Verification items for the finished model (mm, model axes). A direction names the side the tool comes from. Coordinates: 2 decimals unless noted, no trailing zeros. Order: outer loops, then holes, each group sorted by start corner. A loop starts at its lowest first (then second) coordinate and runs counter-clockwise, first axis right, second up. Notation, with made-up numbers: (47, -22.5) -> (105, -22.5) arc R34 ccw to (105, 11.5) -> close; hole circle Ø9 at (-25.5, 41). An arc over 180 degrees is marked (long way). Write each question's results on one line, items separated by ' | '. Start each with the question number.
(1) Go/stop test with flat-tipped pins: pin 1 (1 mm diameter, centred on x = -0.5, z = -1.5, fed in from +Y); pin 2 (11.5 mm diameter, centred on x = 0, z = 0, fed in from -Y); pin 3 (5 mm diameter, centred on x = 6, y = -2, fed in from +Z); pin 4 (5 mm diameter, centred on y = -3.5, z = 2.5, fed in from +X). Record where each tip stops, or that it passes through.
(2) Cross-section at A-A on y = -7.25. Enter the section's corners in (x, z).
(3) Cross-section at C-C on x = 1. Enter the section's corners in (y, z), and give its area (3 significant figures).
(4) Cross-section at B-B on z = 0. Enter the section's corners in (x, y).
(5) Cross-section at D-D on y = -0.25. Enter the section's corners in (x, z), and give its area (3 significant figures).
(6) Thickness scan on probe 1 along Z at (x, y) = (0, 0.1); probe 2 along X at (y, z) = (-7.5, -1.5); probe 3 along Z at (x, y) = (3.5, -5). Record the ranges inside material, lowest first. Write a range as [from, to].
(7) Draft check along X on faces 1 (the flat face through (-14.5, -10.3, 10.4)), 2 (the flat face through (-17.27, -5.48, 5.78)), 3 (the flat face through (8, -0.8, -4)). Enter one of: +X half, -X half, draft (parallel to the pull), parting line (faces both ways), or undercut.
(8) Set-up check for faces 4 (the flat face through (10.58, -5.48, 14.83)), 5 (the cylindrical face through (-6.944, -5.617, -5.324)), 6 (the flat face through (-10.834, -5.483, 14.641)): record each of +Z, -Z, +X, -X, +Y, -Y from which the full face is reachable in a straight line by a thin tool's end or side.
Solid Edge part; units mm, degrees
sketch "Sketch1" plane through (0, 0, 0) normal (0, -1, 0) x (1, 0, 0)
  circle A0 centre (0, 0) radius 19
extrude "Protrusion1" add sketch "Sketch1" along normal mid plane 1.6
sketch "Sketch2" plane through (0, -0.8, 0) normal (0, -1, 0) x (1, 0, 0)
  line L0 (16.5947, -5.2323) -> (18.1683, -5.7284)
  arc A0 (18.1683, 5.7284) -> (18.1683, -5.7284) centre (0, 0) cw
  line L1 (16.5947, 5.2323) -> (18.1683, 5.7284)
  arc A1 (16.5947, 5.2323) -> (16.5947, -5.2323) centre (0, 0) cw
extrude "Protrusion2" add sketch "Sketch2" along normal blind 9.5
pattern_circular "Pattern1" count 5 over 360 about axis through (0, -0.8, 0) along (0, 1, 0) of "Protrusion2"
sketch "Sketch3" plane through (-14.2263, -10.3, -10.4272) normal (0, -1, 0) x (1, 0, 0)
  circle A0 centre (14.2263, 10.4272) radius 8.75
extrude "Protrusion7" add sketch "Sketch3" against normal up to next
sketch "Sketch4" plane through (-0.4408, -0.8, 0) normal (0, -1, 0) x (1, 0, 0)
  circle A0 centre (0.4408, 0) radius 7.15
extrude "Cutout1" cut sketch "Sketch4" along normal through all
sketch "Sketch5" plane through (0, -0.8, 0) normal (0, -1, 0) x (1, 0, 0)
  circle A0 centre (0, 0) radius 3.25
extrude "Cutout2" cut sketch "Sketch5" against normal through all
properties part number "C-101-1" material "STEEL, GALVANIZED"
Results are:
1) pin 1: passes through | pin 2: stops at y = -0.8 | pin 3: stops at z = 18.73 | pin 4: stops at x = 19.05
2) outline: (-18.07, -6.04) arc R19.05 ccw to (-11.33, -15.31) -> (-10.35, -13.99) arc R17.4 cw to (-16.5, -5.52) -> close; (-18.07, 6.04) -> (-16.5, 5.52) arc R17.4 cw to (-10.35, 13.99) -> (-11.33, 15.31) arc R19.05 ccw to start; circle Ø17.5 at (0, 0); (0.15, -17.4) -> (0.17, -19.05) arc R19.05 ccw to (11.06, -15.51) -> (10.1, -14.17) arc R17.4 cw to start; (0.15, 17.4) arc R17.4 cw to (10.1, 14.17) -> (11.06, 15.51) arc R19.05 ccw to (0.17, 19.05) -> close; (16.59, -5.23) -> (18.17, -5.73) arc R19.05 ccw to (18.17, 5.73) -> (16.59, 5.23) arc R17.4 cw to start; hole circle Ø14.3 at (0, 0)
3) outline: (-10.3, -19.02) -> (-0.8, -19.02) -> (-0.8, -18.97) -> (0.8, -18.97) -> (0.8, -3.09) -> (-0.8, -3.09) -> (-0.8, -7.08) -> (-10.3, -7.08) -> (-10.3, -8.69) -> (-0.8, -8.69) -> (-0.8, -17.37) -> (-10.3, -17.37) -> close; (-10.3, 7.08) -> (-0.8, 7.08) -> (-0.8, 3.09) -> (0.8, 3.09) -> (0.8, 18.97) -> (-0.8, 18.97) -> (-0.8, 19.02) -> (-10.3, 19.02) -> (-10.3, 17.37) -> (-0.8, 17.37) -> (-0.8, 8.69) -> (-10.3, 8.69) -> close | area: 113 mm2
4) outline: (-19, -0.8) -> (-8.75, -0.8) -> (-8.75, -10.3) -> (-7.15, -10.3) -> (-7.15, -0.8) -> (-3.25, -0.8) -> (-3.25, 0.8) -> (-19, 0.8) -> close; (3.25, -0.8) -> (7.15, -0.8) -> (7.15, -10.3) -> (8.75, -10.3) -> (8.75, -0.8) -> (17.4, -0.8) -> (17.4, -10.3) -> (19.05, -10.3) -> (19.05, -0.8) -> (19, -0.8) -> (19, 0.8) -> (3.25, 0.8) -> close
5) outline: circle Ø38 at (0, 0); hole circle Ø6.5 at (0, 0) | area: 1,100 mm2
6) probe 1: z = [-19, -3.25], [3.25, 19] | probe 2: x = [-8.62, -6.99], [6.99, 8.62], [17.34, 18.99] | probe 3: z = [-18.73, -17.04], [-8.02, -6.23], [6.23, 8.02], [17.04, 18.73]
7) face 1: draft | face 2: -X half | face 3: undercut
8) face 4: +X, -Y | face 5: -Y | face 6: +Z, -Y
